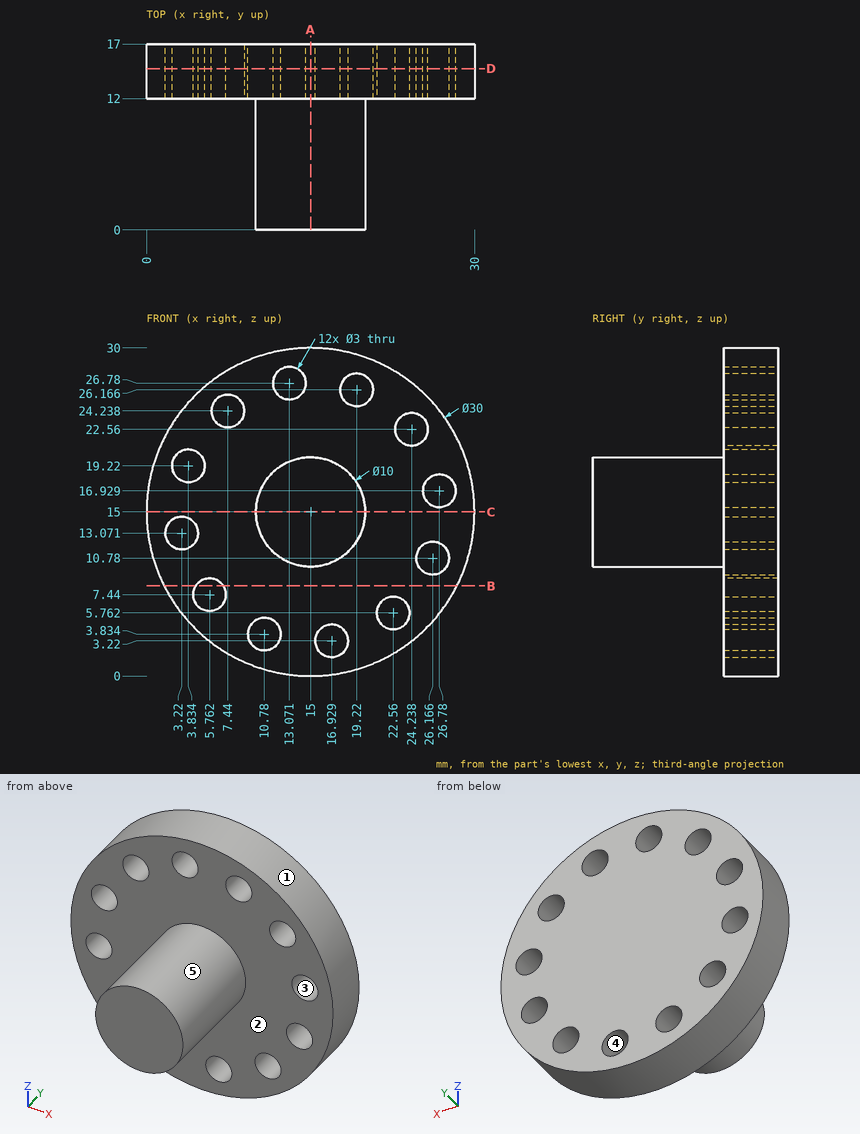
Study the drawing (mm; zero at the part's minimum x, y, z) and answer. A direction names the side the tool comes from. Give positions to 0.01 mm unless a question says otherwise; leave off trailing zeros. Order: outer loops, then holes, each group sorted by start corner. A loop starts at its lowest first (then second) coordinate and runs counter-clockwise, first axis right, second up.
1. Section A-A, the plane x = 15 is taken. Determine the outline of the cut face in (y, z).
Result sheet:
outline: (0, 10) - (12, 10) - (12, 0) - (17, 0) - (17, 30) - (12, 30) - (12, 20) - (0, 20) - close
2. Section B-B, the plane z = 8.25 is taken. Determine the outline of the cut face in (x, y) (1 decimal), and give its area (3 significant figures).
Result sheet:
outline: (1.6, 12) - (4.5, 12) - (4.5, 17) - (1.6, 17) - close; (7, 12) - (28.4, 12) - (28.4, 17) - (7, 17) - close
area: 121 mm2
3. Section D-D, the plane y = 14.75 is taken. Give the number of separate pieces and of enclosed holes in the cut face, and give its area (3 significant figures).
Result sheet:
separate pieces: 1
enclosed holes: 12
area: 622 mm2
4. Each of these flat-tipped pins is pushed along its axis until it touches: P1, Ø2.5, axis at x = 10.78, z = 3.83, coming from the +Y side; P2, Ø5, axis at x = 8, z = 9.5, coming from the -Y side; P3, Ø2, axis at y = 6, z = 15.5, coming from the +X side; P4, Ø1.5, axis at x = 17.5, y = 15, coming from the -Z side. Where does it stop, or does it pass through?
Result sheet:
P1: passes through
P2: stops at y = 12
P3: stops at x = 20
P4: stops at z = 0.1
5. Section C-C, the plane z = 15 is taken. Determine the outline of the cut face in (x, y), and give its area (3 significant figures).
Result sheet:
outline: (0, 12) - (10, 12) - (10, 0) - (20, 0) - (20, 12) - (30, 12) - (30, 17) - (0, 17) - close
area: 270 mm2
6. The mould has two halves that part along Z. Classify the marked faces 1, 2 and 3: released by +Z, released by -Z, zero draft, split by the parting line, or undercut.
Result sheet:
face 1: split by the parting line
face 2: zero draft
face 3: undercut
7. For the marked faces 4 and 5, determine the directions among +Z, -Z, +X, -X, +Y, -Y from which every point of the face is accessible in a straight line to the end or side of a thin tool.
Result sheet:
face 4: +Y, -Y
face 5: -Y
8. Straight lines are drawn through the part: L1, parallel to Y at x = 24, z = 18.5; L2, parallel to X at y = 13, z = 2 (1 decimal); L3, parallel to X at y = 12.5, z = 14 (1 decimal). For each, find the intervals that lie inside material, in ascending order.
Result sheet:
L1: y = 12 to 17
L2: x = 7.5 to 16.1, 17.8 to 22.5
L3: x = 0 to 2, 4.4 to 30
